Design review of the part built by this model. Coordinates are the model's own, in mm. Face numbers are marked on the shaded views. Round coordinates to 2 decimals unless told otherwise and drop trailing zeros. Loops run counter-clockwise (first coordinate to the right, second up) from the corner with the lowest first, then second, coordinate; pieces in that order, holes last. Notation, with made-up numbers: (40, 80) - (77, 80) arc R33 ccw to (77, 116) - close; hole circle Ø1 at (-18.5, -7.75). An arc over 180 degrees is marked (long way). Return JSON: item names as keys, results as strings. Group by question number.
(1) We need section C-C, the plane z = 85. Write out the cut boundary in (x, y).
(2) We need section D-D, the plane x = -10.5. Give the number of separate pieces and of enclosed holes in the cut face, and give its area (3 significant figures).
(3) We need section A-A, the plane y = 0. Write out the cut boundary in (x, z), and give its area (3 significant figures).
(4) We need section B-B, the plane z = 0. Write out the cut boundary in (x, y).
(5) Clearance check with flat-ended pins moving along their axes: pin 1 (5 mm diameter, centred on x = 5.5, y = -51.5, fed in from -Z); pin 2 (8 mm diameter, centred on y = 60.1, z = -60.1, fed in from +X); pin 3 (8 mm diameter, centred on x = 10.5, y = 38.5, fed in from -Z); pin 4 (5 mm diameter, centred on x = -14.5, z = 77.5, fed in from +Y). State where each tip first meets the part, or that it passes through.
(6) Wall thickness on L1, parallel to Y at x = 8.5, z = -73; L2, parallel to Z at x = 4, y = -42; L3, parallel to Y at x = -6, z = 2: over which ranges is each line inside the solid? List them lowest first. Write a range as [from, to].
(7) The part is to be moulded in two halves that separate along Y. For the marked faces 1, 2 and 3, say which applies: pulls with the +Y half, pulls with the -Y half, needs draft (parallel to the pull), parting line crosses it, or undercut.
from build123d import *

# Parameters (mm, degrees)
SKETCH1_W                       = 38
SKETCH1_H                       = 35
SKETCH2_R                       = 6.5
CUT_EXTRUDE1_DEPTH              = 154.277526076
CIRPATTERN1_COUNT               = 5
CIRPATTERN1_ANGLE               = 60
CIRPATTERN1_THE_OTHER_WAY_COUNT = 5
CIRPATTERN1_THE_OTHER_WAY_ANGLE = 60
MIRROR1_COPY_1_SKETCH_R         = 6.5
MIRROR1_COPY_1_DEPTH            = 154.277526076
MIRROR1_COPY_2_SKETCH_R         = 6.5
MIRROR1_COPY_2_DEPTH            = 154.277526076
MIRROR1_COPY_3_SKETCH_R         = 6.5
MIRROR1_COPY_3_DEPTH            = 154.277526076
MIRROR1_COPY_4_SKETCH_R         = 6.5
MIRROR1_COPY_4_DEPTH            = 154.277526076
MIRROR1_COPY_5_SKETCH_R         = 6.5
MIRROR1_COPY_5_DEPTH            = 154.277526076
MIRROR1_COPY_6_SKETCH_R         = 6.5
MIRROR1_COPY_6_DEPTH            = 154.277526076
MIRROR1_COPY_7_SKETCH_R         = 6.5
MIRROR1_COPY_7_DEPTH            = 154.277526076
MIRROR1_COPY_8_SKETCH_R         = 6.5
MIRROR1_COPY_8_DEPTH            = 154.277526076
CHAMFER1_SIZE                   = 3


with BuildPart() as part:
    # Sketch1 → Revolve1 (revolve)
    with BuildSketch(Plane.XY, mode=Mode.PRIVATE) as revolve1_sk:
        with Locations((0, 87.5)):
            Rectangle(SKETCH1_W, SKETCH1_H)
    revolve(revolve1_sk.sketch.rotate(Axis((0, 0, 0), (-1, 0, 0)), 90), axis=Axis((0, 0, 0), (-1, 0, 0)))

    # Sketch2 → Cut-Extrude1 (cut, through all)
    with BuildSketch(Plane(origin=(19, 0, 0), x_dir=(0, 0, -1), z_dir=(1, 0, 0))):
        with Locations((85, 0)):
            Circle(SKETCH2_R)
    cut_extrude1 = extrude(amount=-CUT_EXTRUDE1_DEPTH, mode=Mode.SUBTRACT)

    # CirPattern1: Cut-Extrude1 ×5 about axis
    cirpattern1_axis = Axis((0, 0, 0), (1, 0, 0))
    for i in range(1, CIRPATTERN1_COUNT):
        add(cut_extrude1.rotate(cirpattern1_axis, i * CIRPATTERN1_ANGLE / (CIRPATTERN1_COUNT - 1)), mode=Mode.SUBTRACT)

    # CirPattern1 the other way: Cut-Extrude1 ×5 about axis
    cirpattern1_the_other_way_axis = Axis((0, 0, 0), (-1, 0, 0))
    for i in range(1, CIRPATTERN1_THE_OTHER_WAY_COUNT):
        add(cut_extrude1.rotate(cirpattern1_the_other_way_axis, i * CIRPATTERN1_THE_OTHER_WAY_ANGLE / (CIRPATTERN1_THE_OTHER_WAY_COUNT - 1)), mode=Mode.SUBTRACT)

    # Mirror1: Cut-Extrude1 across plane
    add(cut_extrude1.mirror(Plane.XY), mode=Mode.SUBTRACT)

    # Mirror1 copy 1 sketch → Mirror1 copy 1 (cut, through all)
    with BuildSketch(Plane(origin=(19, 0, 0), x_dir=(0, 0.2588190451025214, 0.9659258262890681), z_dir=(1, 0, 0))):
        with Locations((85, 0)):
            Circle(MIRROR1_COPY_1_SKETCH_R)
    extrude(amount=-MIRROR1_COPY_1_DEPTH, mode=Mode.SUBTRACT)

    # Mirror1 copy 2 sketch → Mirror1 copy 2 (cut, through all)
    with BuildSketch(Plane(origin=(19, 0, 0), x_dir=(0, 0.5000000000000011, 0.866025403784438), z_dir=(1, 0, 0))):
        with Locations((85, 0)):
            Circle(MIRROR1_COPY_2_SKETCH_R)
    extrude(amount=-MIRROR1_COPY_2_DEPTH, mode=Mode.SUBTRACT)

    # Mirror1 copy 3 sketch → Mirror1 copy 3 (cut, through all)
    with BuildSketch(Plane(origin=(19, 0, 0), x_dir=(0, 0.7071067811865488, 0.7071067811865462), z_dir=(1, 0, 0))):
        with Locations((85, 0)):
            Circle(MIRROR1_COPY_3_SKETCH_R)
    extrude(amount=-MIRROR1_COPY_3_DEPTH, mode=Mode.SUBTRACT)

    # Mirror1 copy 4 sketch → Mirror1 copy 4 (cut, through all)
    with BuildSketch(Plane(origin=(19, 0, 0), x_dir=(0, 0.8660254037844399, 0.4999999999999978), z_dir=(1, 0, 0))):
        with Locations((85, 0)):
            Circle(MIRROR1_COPY_4_SKETCH_R)
    extrude(amount=-MIRROR1_COPY_4_DEPTH, mode=Mode.SUBTRACT)

    # Mirror1 copy 5 sketch → Mirror1 copy 5 (cut, through all)
    with BuildSketch(Plane(origin=(19, 0, 0), x_dir=(0, -0.2588190451025214, 0.9659258262890681), z_dir=(1, 0, 0))):
        with Locations((85, 0)):
            Circle(MIRROR1_COPY_5_SKETCH_R)
    extrude(amount=-MIRROR1_COPY_5_DEPTH, mode=Mode.SUBTRACT)

    # Mirror1 copy 6 sketch → Mirror1 copy 6 (cut, through all)
    with BuildSketch(Plane(origin=(19, 0, 0), x_dir=(0, -0.5000000000000011, 0.866025403784438), z_dir=(1, 0, 0))):
        with Locations((85, 0)):
            Circle(MIRROR1_COPY_6_SKETCH_R)
    extrude(amount=-MIRROR1_COPY_6_DEPTH, mode=Mode.SUBTRACT)

    # Mirror1 copy 7 sketch → Mirror1 copy 7 (cut, through all)
    with BuildSketch(Plane(origin=(19, 0, 0), x_dir=(0, -0.7071067811865488, 0.7071067811865462), z_dir=(1, 0, 0))):
        with Locations((85, 0)):
            Circle(MIRROR1_COPY_7_SKETCH_R)
    extrude(amount=-MIRROR1_COPY_7_DEPTH, mode=Mode.SUBTRACT)

    # Mirror1 copy 8 sketch → Mirror1 copy 8 (cut, through all)
    with BuildSketch(Plane(origin=(19, 0, 0), x_dir=(0, -0.8660254037844399, 0.4999999999999978), z_dir=(1, 0, 0))):
        with Locations((85, 0)):
            Circle(MIRROR1_COPY_8_SKETCH_R)
    extrude(amount=-MIRROR1_COPY_8_DEPTH, mode=Mode.SUBTRACT)

    # Chamfer1
    chamfer1_edges = [part.edges().sort_by_distance(p)[0] for p in [
        (19, 0, 70),
        (-19, 0, 70),
    ]]
    chamfer(chamfer1_edges, length=CHAMFER1_SIZE)


solid = part.part
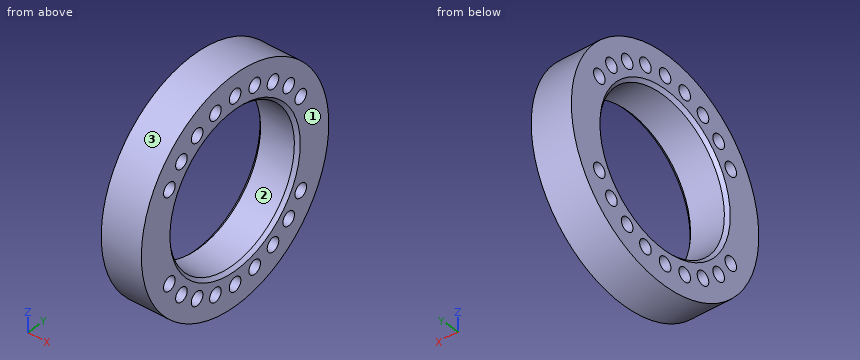
Solutions:
{
 "1": {"outline": "(-19, -61.64) - (19, -61.64) - (19, -27.82) - (-19, -27.82) - close; (-19, -16.18) - (19, -16.18) - (19, -6.5) - (-19, -6.5) - close; (-19, 6.5) - (19, 6.5) - (19, 16.18) - (-19, 16.18) - close; (-19, 27.82) - (19, 27.82) - (19, 61.64) - (-19, 61.64) - close"},
 "2": {"separate pieces": "1", "enclosed holes": "19", "area": "16,900 mm^2"},
 "3": {"outline": "(-19, -105) - (19, -105) - (19, -91.5) - (-19, -91.5) - close; (-19, -78.5) - (19, -78.5) - (19, -73) - (16, -70) - (-16, -70) - (-19, -73) - close; (-19, 73) - (-16, 70) - (16, 70) - (19, 73) - (19, 78.5) - (-19, 78.5) - close; (-19, 91.5) - (19, 91.5) - (19, 105) - (-19, 105) - close", "area": "1,650 mm^2"},
 "4": {"outline": "(-19, -105) - (19, -105) - (19, -73) - (16, -70) - (-16, -70) - (-19, -73) - close; (-19, 73) - (-16, 70) - (16, 70) - (19, 73) - (19, 105) - (-19, 105) - close"},
 "5": {"pin 1": "z = -92.87", "pin 2": "through", "pin 3": "z = -99.17", "pin 4": "y = 73.48"},
 "6": {"L1": "[-75.47, -48.97], [-36.03, 36.03], [48.97, 75.47]", "L2": "[-96.23, -80.09], [-67.13, -56], [56, 67.13], [80.09, 96.23]", "L3": "[-104.98, -69.97], [69.97, 104.98]"},
 "7": {"face 1": "needs draft", "face 2": "undercut", "face 3": "parting line crosses it"}
}
